```python
from build123d import *

# Parameters (mm, degrees)
EXTRUDE_1_DEPTH     = 1.2
CUT_EXTRUDE_START   = -1.2
CUT_EXTRUDE_1_DEPTH = 1.2
SKETCH_4_R          = 0.3
EXTRUDE_2_DEPTH     = 0.3
SKETCH_5_W          = 8.574992792
SKETCH_5_H          = 35.59001433
EXTRUDE_3_DEPTH     = 0.6


# Read off the part's stored shape, not the designer's step: Вырез-Вытянуть-Тонкостенный1
with BuildPart() as part:
    # Эскиз1 → Бобышка-Вытянуть1 (new body)
    with BuildSketch(Plane.XY):
        with BuildLine():
            Line((-5.154205728, -20.72997941), (-0.373828409, -24.299606142))
            Line((-0.373828409, -24.299606142), (7.292363911, -18.166652286))
            Line((7.292363911, -18.166652286), (5.355661958, 11.708005491))
            Line((5.355661958, 11.708005491), (0.043580434, 24.299606142))
            Line((0.043580434, 24.299606142), (-0.335864947, 24.169962303))
            add(Edge.make_bspline(
                [(-0.335864947, 24.169962303), (-0.915680869, 23.882560356), (-2.036028517, 23.32722877), (-3.511970223, 22.237099766), (-4.75482851, 21.003209681), (-5.762815681, 19.609778776), (-6.510522146, 18.041460832), (-7.00511156, 16.321943976), (-7.292363911, 14.445670921), (-7.266146832, 13.148358332), (-7.252515423, 12.473828633)],
                knots=[0, 0, 0, 0, 0.133243547, 0.257459461, 0.376453369, 0.49320762, 0.610289886, 0.732843248, 0.86109349, 1, 1, 1, 1], degree=3))
            Line((-7.252515423, 12.473828633), (-5.154205728, -20.72997941))
        make_face()
    extrude(amount=EXTRUDE_1_DEPTH)

    # Вырез-Вытянуть-Тонкостенный1 outline → Вырез-Вытянуть-Тонкостенный1 (cut)
    with BuildSketch(Plane.XY.offset(1.2).offset(CUT_EXTRUDE_START)):
        with BuildLine():
            Line((0.043580434, 24.299606142), (-0.335864947, 24.169962303))
            add(Edge.make_bspline(
                [(-0.335864947, 24.169962303), (-0.915680869, 23.882560356), (-2.036028517, 23.32722877), (-3.511970223, 22.237099766), (-4.75482851, 21.003209681), (-5.762815681, 19.609778776), (-6.510522146, 18.041460832), (-7.00511156, 16.321943976), (-7.292363911, 14.445670921), (-7.266146832, 13.148358332), (-7.252515423, 12.473828633)],
                knots=[0, 0, 0, 0, 0.133243547, 0.257459461, 0.376453369, 0.49320762, 0.610289886, 0.732843248, 0.86109349, 1, 1, 1, 1], degree=3))
            Line((-7.252515423, 12.473828633), (-5.154205728, -20.72997941))
            Line((-5.154205728, -20.72997941), (-0.373828409, -24.299606142))
            Line((-0.373828409, -24.299606142), (7.292363911, -18.166652286))
            Line((7.292363911, -18.166652286), (5.355661958, 11.708005491))
            Line((5.355661958, 11.708005491), (0.043580434, 24.299606142))
        make_face()
        with BuildLine():
            add(Edge.make_bspline(
                [(-0.181718189, 23.79992617), (-0.707013415, 23.539538063), (-1.232077833, 23.278807084), (-2.230510803, 22.680549291), (-2.702172016, 22.340486172), (-3.596295179, 21.58727288), (-4.022133554, 21.170752521), (-4.785274575, 20.282262055), (-5.126061609, 19.808572418), (-5.567321736, 19.047557585), (-5.703329339, 18.784315196), (-5.950182465, 18.247397148), (-6.060575566, 17.974952319), (-6.35630443, 17.146776614), (-6.507229216, 16.580522405), (-6.739435456, 15.426716133), (-6.817026677, 14.83956809), (-6.876685102, 13.667024978), (-6.864657606, 13.078754602), (-6.852770472, 12.490490929)],
                knots=[0, 0, 0, 0, 0.125, 0.125, 0.25, 0.25, 0.375, 0.375, 0.5, 0.5, 0.5625, 0.5625, 0.625, 0.625, 0.75, 0.75, 0.875, 0.875, 1, 1, 1, 1], degree=3))
            Line((-0.181718189, 23.79992617), (-0.180003158, 23.800512138))
            Line((-0.180003158, 23.800512138), (4.960868317, 11.614742715))
            Line((4.960868317, 11.614742715), (6.879717061, -17.984519827))
            Line((6.879717061, -17.984519827), (-0.382255806, -23.794098121))
            Line((-0.382255806, -23.794098121), (-4.766668047, -20.520148369))
            Line((-4.766668047, -20.520148369), (-6.852770472, 12.490490929))
        make_face(mode=Mode.SUBTRACT)
    extrude(amount=CUT_EXTRUDE_1_DEPTH, mode=Mode.SUBTRACT)

    # Эскиз4 → Бобышка-Вытянуть2 (add)
    with BuildSketch(Plane(origin=(-6.03931721, -0.38165375, 0), x_dir=(0, 0, 1), z_dir=(-0.9980091663650418, -0.06306904035542692, 0))):
        with Locations(Location((0.6, -19.578666988, 0), (0, 0, 270))):
            Circle(SKETCH_4_R)
        with Locations(Location((0.6, -8.978666988, 0), (0, 0, 270))):
            Circle(SKETCH_4_R)
        with Locations(Location((0.6, 1.621333012, 0), (0, 0, 270))):
            Circle(SKETCH_4_R)
        with Locations(Location((0.6, 12.221333012, 0), (0, 0, 270))):
            Circle(SKETCH_4_R)
    extrude(amount=EXTRUDE_2_DEPTH)

    # Эскиз5 → Бобышка-Вытянуть3 (add)
    with BuildSketch(Plane(origin=(-6.33871996, -0.400574462, 0), x_dir=(0, 0, 1), z_dir=(-0.9980091663650418, -0.06306904035542692, 0))):
        with Locations((0.334402878, -3.441718967)):
            Rectangle(SKETCH_5_W, SKETCH_5_H)
    extrude(amount=EXTRUDE_3_DEPTH)


solid = part.part
```
The model under review builds one solid part; all positions refer to its coordinate system, in mm. Round coordinates to 2 decimals unless told otherwise and drop trailing zeros. Order: outer loops, then holes, each group sorted by start corner. A loop starts at its lowest first (then second) coordinate and runs counter-clockwise, first axis right, second up. Notation, with made-up numbers: M -13,31 L 6,31 A15 cw 6,40 Z; hole C 75.25,1 d2. An arc over 180 degrees is marked long. Use a Markdown table: item, result.
1) Consider section C-C (y = -4.5). Write out the cut boundary in (x, z), then the cut area to 3 significant figures.
Report:
| item | result |
|---|---|
| outline | M -6.68,-3.95 L -6.08,-3.95 L -6.08,4.62 L -6.68,4.62 Z; M -5.78,0 L 6.01,0 L 6.01,1.2 L -5.78,1.2 Z |
| area | 19.3 mm^2 |
2) Insertion check: pin 1 (3 mm diameter, centred on y = 10, z = 1, fed in from -X); pin 2 (4 mm diameter, centred on x = 4.5, y = -16.5, fed in from -Z); pin 3 (2 mm diameter, centred on x = -1, y = -6.5, fed in from +Z); pin 4 (4 mm diameter, centred on x = -2, z = -2.5, fed in from +Y). Each pin has a flat end and moves straight along its axis. Give the tip position at first contact, or say it passes through.
Report:
| item | result |
|---|---|
| pin 1 | x = -7.69 |
| pin 2 | z = 0 |
| pin 3 | z = 1.2 |
| pin 4 | through |
3) Wall thickness on line 1 along Z through (x, y) = (3.5, 0); line 2 along X through (y, z) = (-1, 1); line 3 along X through (y, z) = (-19.5, 1.25): over which ranges is each line inside the solid? List them lowest first. Write a range as [from, to].
Report:
| item | result |
|---|---|
| line 1 | [0, 1.2] |
| line 2 | [-6.9, -6.3], [-6, 5.78] |
| line 3 | [-5.73, -5.13] |
4) Consider section A-A (y = 3). Write out the cut boundary in (x, z), then the cut area to 3 significant figures.
Report:
| item | result |
|---|---|
| outline | M -7.15,-3.95 L -6.55,-3.95 L -6.55,4.62 L -7.15,4.62 Z; M -6.25,0 L 5.52,0 L 5.52,1.2 L -6.25,1.2 Z |
| area | 19.3 mm^2 |
5) Consider section B-B (z = -2). Write out the cut boundary in (x, y).
Report:
| item | result |
|---|---|
| outline | M -7.84,13.89 L -5.6,-21.63 L -5,-21.6 L -7.24,13.92 Z |
6) Draft analysis for pull direction X (two halves, no side actions). For faces 1 (the face through (-6.4, -4.1, -3.953)), 2 (the face through (3.3, -20.85, 0.59)), 3 (the face through (-2.544, -22.18, 0.592)), state which applies: released by +X, released by -X, zero draft, split by the parting line, or undercut.
Report:
| item | result |
|---|---|
| face 1 | zero draft |
| face 2 | released by +X |
| face 3 | undercut |
7) Consider section D-D (x = 5.5). Write out the cut boundary in (y, z).
Report:
| item | result |
|---|---|
| outline | M -19.09,0 L 3.3,0 L 3.3,1.2 L -19.09,1.2 Z |
